Autodesk Inventor part; units mm, degrees
ref_plane "YZ Plane" through (0, 0, 0) normal (1, 0, 0) x (0, 1, 0)
ref_plane "XZ Plane" through (0, 0, 0) normal (0, 1, 0) x (-1, 0, 0)
ref_plane "XY Plane" through (0, 0, 0) normal (0, 0, 1) x (1, 0, 0)
sketch "Sketch1" plane through (0, 0, 0) normal (0, 0, 1) x (1, 0, 0)
  line L0 (5.5291, -4.6499) -> (-42.4709, -4.6499)
  line L1 (-42.4709, -4.6499) -> (-42.4709, -52.6499)
  line L2 (-42.4709, -52.6499) -> (5.5291, -52.6499)
  line L3 (5.5291, -52.6499) -> (5.5291, -4.6499)
  line L4 (5.5291, -4.6499) -> (5.5291, -8.6499)
  line L5 (5.5291, -8.6499) -> (1.5291, -8.6499)
  circle A0 centre (1.5291, -8.6499) radius 1.5
  line L6 (-42.4709, -4.6499) -> (-42.4709, -8.6499)
  line L7 (-42.4709, -8.6499) -> (-32.4709, -8.6499)
  circle A1 centre (-32.4709, -8.6499) radius 1.5
  line L8 (5.5291, -52.6499) -> (5.5291, -42.6499)
  line L9 (5.5291, -42.6499) -> (1.5291, -42.6499)
  circle A2 centre (1.5291, -42.6499) radius 1.5
  point P0 (0, 0)
  dimension "d0" = 48
  dimension "d1" = 48
  dimension "d2" = 4
  dimension "d3" = 4
  dimension "d4" = 3
  dimension "d5" = 4
  dimension "d6" = 10
  dimension "d7" = 3
  dimension "d8" = 10
  dimension "d9" = 4
  dimension "d10" = 3
extrude "Extrusion1" add sketch "Sketch1" along normal blind 2
properties part number "contorller kort"
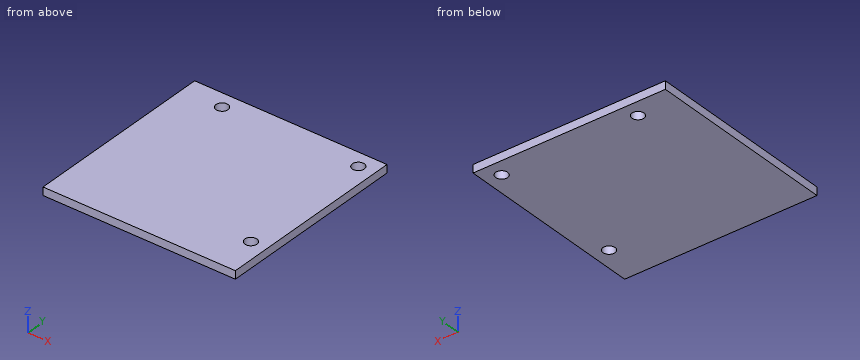
The model under review builds one solid part; all positions refer to its coordinate system, in mm. Round coordinates to 2 decimals unless told otherwise and drop trailing zeros. Order: outer loops, then holes, each group sorted by start corner. A loop starts at its lowest first (then second) coordinate and runs counter-clockwise, first axis right, second up. Notation, with made-up numbers: (51, -15) -> (75, -15) arc R18 ccw to (75, 7) -> close; hole circle Ø1 at (42.25, -10). An arc over 180 degrees is marked (long way). Use CSV: the item, a comma, the result in double quotes. Start each with the question number.
(1) Wall thickness on probe 1 along X at (y, z) = (-7.5, 0.95); probe 2 along X at (y, z) = (-42, 1.65): over which ranges is each line inside the solid? List them lowest first. Write a range as from..to.
(2) Consider section A-A on y = -42. Write out the cut boundary in (x, z), and give its area (3 significant figures).
(3) Insertion check: pin 1 (2.5 mm diameter, centred on x = -32.47, y = -8.65, fed in from +Z). The pin has a flat end and moves straight along its axis. Give the tip position at first contact, or say it passes through.
Responses:
1,probe 1,"-42.47..-33.43, -31.51..0.57, 2.49..5.53"
1,probe 2,"-42.47..0.18, 2.88..5.53"
2,outline,"(-42.47, 0) -> (0.18, 0) -> (0.18, 2) -> (-42.47, 2) -> close; (2.88, 0) -> (5.53, 0) -> (5.53, 2) -> (2.88, 2) -> close"
2,area,"90.6 mm²"
3,pin 1,"through"
